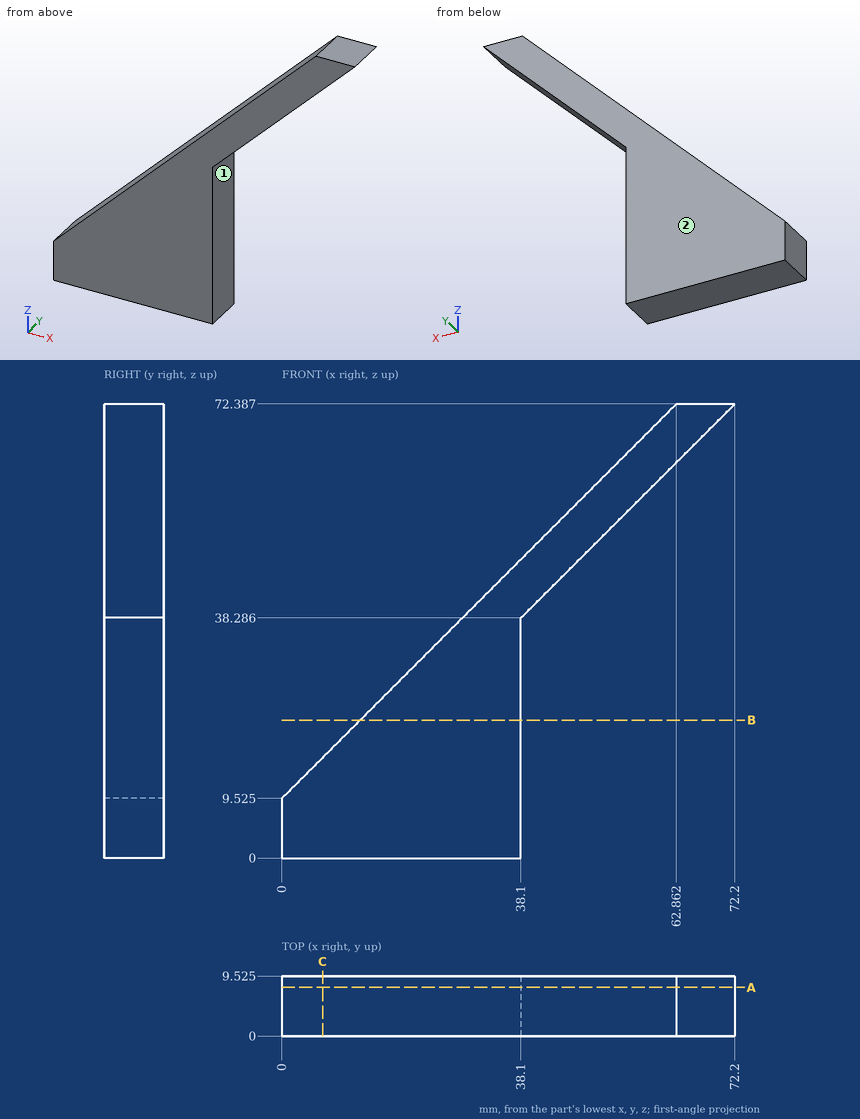
Study the drawing (mm; zero at the part's minimum x, y, z) and answer. A direction names the side the tool comes from. Coordinates: 2 decimals unless noted, no trailing zeros. Write each loop counter-clockwise with the first axis right and the second up, starting at its lowest first coordinate (ties: lowest second). Pieces come first, ordered by that corner, then holes. Notation, with made-up numbers: (65.5, -15.5) - (85.5, -15.5) arc R24 ccw to (85.5, 0.5) - close; hole circle Ø4 at (-17, 72). An arc over 180 degrees is marked (long way). Answer as a JSON object with one key per item and string values. Group by question number.
1. A cutting plane is placed at A-A (y = 7.75). Determine the outline of the cut face in (x, z) (1 decimal).
2. A cutting plane is placed at B-B (z = 22). Determine the outline of the cut face in (x, y) (1 decimal).
3. Which of the six approach directions +Z, -Z, +X, -X, +Y, -Y give full straight-line access (tool end or side, diameter ignored) to the marked faces 1 and 2?
4. Consider L1, parallel to X at y = 1, z = 4; L2, parallel to X at y = 1.5, z = 65 (1 decimal); L3, parallel to Z at x = 54, y = 1.5 (1 decimal). Determine where each line is inside the solid, lowest interval first. Write a range as [from, to].
5. Each of these flat-tipped pins is pushed along its axis until it touches: P1, Ø1, axis at y = 8, z = 29.5, coming from the -X side (1 decimal); P2, Ø5, axis at x = 9.5, z = 25.5, coming from the -Y side; P3, Ø2, axis at x = 57, y = 1, coming from the -Z side (1 decimal). Where does it stop, or does it pass through?
6. A cutting plane is placed at C-C (x = 6.5). Determine the outline of the cut face in (y, z) (1 decimal), plus the area to 3 significant figures.
Worked out:
{
 "1": {"outline": "(0, 0) - (38.1, 0) - (38.1, 38.3) - (72.2, 72.4) - (62.9, 72.4) - (0, 9.5) - close"},
 "2": {"outline": "(12.5, 0) - (38.1, 0) - (38.1, 9.5) - (12.5, 9.5) - close"},
 "3": {"face 1": "-Z, +X, +Y, -Y", "face 2": "+Z, -Z, +X, -X, +Y"},
 "4": {"L1": "x = [0, 38.1]", "L2": "x = [55.5, 64.8]", "L3": "z = [54.2, 63.5]"},
 "5": {"P1": "stops at x = 19.5", "P2": "passes through", "P3": "stops at z = 56.2"},
 "6": {"outline": "(0, 0) - (9.5, 0) - (9.5, 16) - (0, 16) - close", "area": "153 mm²"}
}
